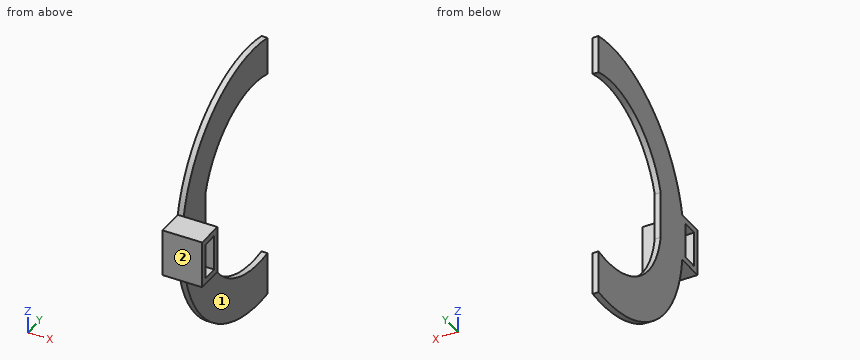
```python
from build123d import *

# Parameters (mm, degrees)
SKETCH1_W           = 24
SKETCH1_H           = 14
SKETCH1_W_2         = 18
SKETCH1_H_2         = 8
BOSS_EXTRUDE1_DEPTH = 20
SKETCH3_W           = 3
SKETCH3_H           = 24
BOSS_EXTRUDE2_DEPTH = 20
BOSS_EXTRUDE4_DEPTH = 3


with BuildPart() as part:
    # Sketch1 → Boss-Extrude1 (new body)
    with BuildSketch(Plane(origin=(0, 0, 0), x_dir=(0, 0, -1), z_dir=(1, 0, 0))):
        with Locations((12, 7)):
            Rectangle(SKETCH1_W, SKETCH1_H)
        with Locations((12, 7)):
            Rectangle(SKETCH1_W_2, SKETCH1_H_2, mode=Mode.SUBTRACT)
    extrude(amount=BOSS_EXTRUDE1_DEPTH)

    # Sketch3 → Boss-Extrude2 (add)
    with BuildSketch(Plane(origin=(0, 14, 0), x_dir=(1, 0, 0), z_dir=(0, 1, 0))):
        with Locations((1.5, 12)):
            Rectangle(SKETCH3_W, SKETCH3_H)
    extrude(amount=BOSS_EXTRUDE2_DEPTH)

    # Sketch5 → Boss-Extrude4 (add)
    with BuildSketch(Plane(origin=(3, 0, 0), x_dir=(0, 0, -1), z_dir=(1, 0, 0))):
        with BuildLine():
            Line((-49.592274582, 91.528999548), (-30.16014503, 91.528999548))
            ThreePointArc((-30.16014503, 91.528999548), (-26.994718436, 56.518129217), (0, 34))
            Line((0, 34), (0, 14))
            ThreePointArc((0, 14), (-40.852918836, 42.493603413), (-49.592274582, 91.528999548))
        make_face()
        with BuildLine():
            Line((65.909693645, 91.528999548), (87.792134304, 91.528999548))
            ThreePointArc((87.792134304, 91.528999548), (71.952848697, 39.552716173), (24, 14))
            Line((24, 14), (24, 34))
            ThreePointArc((24, 34), (56.869492744, 54.084718023), (65.909693645, 91.528999548))
        make_face()
    extrude(amount=-BOSS_EXTRUDE4_DEPTH)


solid = part.part
```
Here's how the part is built. I have some questions about the finished solid (model axes, mm). Face numbers are marked on the shaded views. A direction names the side the tool comes from. Coordinates: 2 decimals unless noted, no trailing zeros. Write each loop counter-clockwise with the first axis right and the second up, starting at its lowest first coordinate (ties: lowest second). Pieces come first, ordered by that corner, then holes. Notation, with made-up numbers: (-11, 82.25) -> (-3, 82.25) arc R25 cw to (-3, 109.25) -> close; hole circle Ø1 at (-12, -33.75). An arc over 180 degrees is marked (long way). Use a Markdown table: item, result. Add a question column.
(1) Please list where these lines run through material, in increasing order: line 1 (Y direction, x = 16.75, z = -17); line 2 (X direction, y = 41.5, z = -62); line 3 (Z direction, x = 8.5, y = 13).
(2) For the marked faces 1 and 2, which set-ups out of +Z, -Z, +X, -X, +Y, -Y let a thin tool reach every point of the face, with its end or its side?
(3) If we section it at B-B, the plane y = 7: Write out the boundary of the cut face in (x, z), and give its area (3 significant figures).
(4) If we section it at A-A, the plane z = -19.5: Write out the boundary of the cut face in (x, y), and give its area (3 significant figures).
(5) I'm going to push flat-ended pins straight in: P1, Ø12, axis at x = 2, z = -43, coming from the -Y side; P2, Ø9, axis at x = 11.5, y = 5.5, coming from the +Z side; P3, Ø1, axis at x = 2.5, y = 77.5, coming from the +Z side; P4, Ø2, axis at y = 27.5, z = 24, coming from the -X side. Where does each tip first touch, or does it pass through?
(6) If we section it at D-D, the plane y = 54: Write out the boundary of the cut face in (x, z), and give its area (3 significant figures).
(7) If we section it at C-C, the plane x = 6: Write out the boundary of the cut face in (y, z).
Outcome:
| question | item | result |
|---|---|---|
| 1 | line 1 | y = 0 to 3, 11 to 14 |
| 1 | line 2 | x = 0 to 3 |
| 1 | line 3 | z = -24 to 0 |
| 2 | face 1 | +Z, -Z, +X, +Y |
| 2 | face 2 | +Z, -Z, +X, -X, -Y |
| 3 | outline | (0, -24) -> (20, -24) -> (20, -21) -> (0, -21) -> close; (0, -3) -> (20, -3) -> (20, 0) -> (0, 0) -> close |
| 3 | area | 120 mm^2 |
| 4 | outline | (0, 0) -> (20, 0) -> (20, 3) -> (0, 3) -> close; (0, 11) -> (20, 11) -> (20, 14) -> (3, 14) -> (3, 34) -> (0, 34) -> close |
| 4 | area | 180 mm^2 |
| 5 | P1 | stops at y = 16.5 |
| 5 | P2 | stops at z = 0 |
| 5 | P3 | stops at z = 51.11 |
| 5 | P4 | stops at x = 0 |
| 6 | outline | (0, -81.16) -> (3, -81.16) -> (3, -56.81) -> (0, -56.81) -> close; (0, 25.57) -> (3, 25.57) -> (3, 46.69) -> (0, 46.69) -> close |
| 6 | area | 136 mm^2 |
| 7 | outline | (0, -24) -> (14, -24) -> (14, 0) -> (0, 0) -> close; hole (3, -21) -> (11, -21) -> (11, -3) -> (3, -3) -> close |
